from build123d import *

# Parameters (mm, degrees)
BOSS_EXTRUDE1_DEPTH = 50.8
SKETCH2_R           = 3.175
CUT_EXTRUDE1_DEPTH  = 64.5
SKETCH3_R           = 5.08
CUT_EXTRUDE2_DEPTH  = 19.05


with BuildPart() as part:
    # Sketch1 → Boss-Extrude1 (new body)
    with BuildSketch(Plane.XY):
        with BuildLine():
            Line((0, 101.6), (0, 114.3))
            ThreePointArc((0, 114.3), (-63.5, 50.8), (0, -12.7))
            Line((0, -12.7), (0, 0))
            ThreePointArc((0, 0), (-50.8, 50.8), (0, 101.6))
        make_face()
    extrude(amount=BOSS_EXTRUDE1_DEPTH)

    # Sketch2 → Cut-Extrude1 (cut, through all)
    with BuildSketch(Plane(origin=(0, 0, 0), x_dir=(0, 0, -1), z_dir=(1, 0, 0))):
        with Locations((-44.45, 107.95)):
            Circle(SKETCH2_R)
        with Locations((-6.35, 107.95)):
            Circle(SKETCH2_R)
        with Locations((-6.35, -6.35)):
            Circle(SKETCH2_R)
        with Locations((-44.45, -6.35)):
            Circle(SKETCH2_R)
    extrude(amount=-CUT_EXTRUDE1_DEPTH, mode=Mode.SUBTRACT)

    # Sketch3 → Cut-Extrude2 (cut)
    with BuildSketch(Plane(origin=(-38.1, 0, 0), x_dir=(0, 0, -1), z_dir=(1, 0, 0))):
        with Locations((-44.45, 107.95)):
            Circle(SKETCH3_R)
        with Locations((-6.35, 107.95)):
            Circle(SKETCH3_R)
        with Locations((-6.35, -6.35)):
            Circle(SKETCH3_R)
        with Locations((-44.45, -6.35)):
            Circle(SKETCH3_R)
    extrude(amount=CUT_EXTRUDE2_DEPTH, mode=Mode.SUBTRACT)


solid = part.part
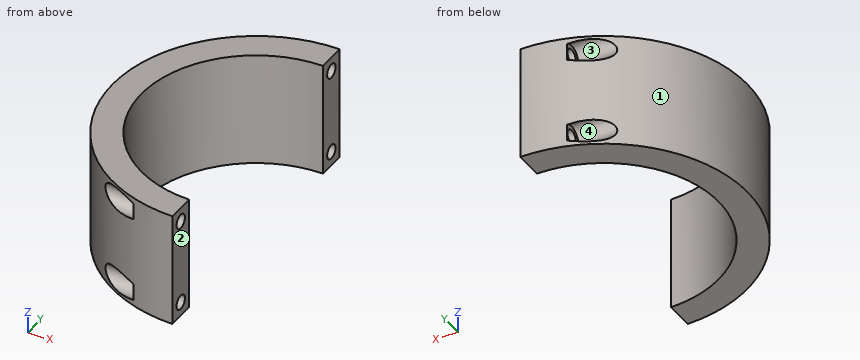
Design review of the part built by this model. Coordinates are the model's own, in mm. Face numbers are marked on the shaded views. Give positions to 0.01 mm unless a question says otherwise; leave off trailing zeros. Order: outer loops, then holes, each group sorted by start corner. A loop starts at its lowest first (then second) coordinate and runs counter-clockwise, first axis right, second up. Notation, with made-up numbers: (30.5, 44.25) - (53.5, 44.25) arc R9 ccw to (53.5, 59.25) - close; hole circle Ø1 at (-16, 9.5). An arc over 180 degrees is marked (long way). Use CSV: the item, a comma, the result in double quotes. Start each with the question number.
Q1. For line 1 (Z direction, x = -25, y = -6); line 2 (Y direction, x = -7.25, z = 44.45) (3 decimals); line 3 (Y direction, x = -13, z = 5), list the stretches that pass through material, from the lowest coordinate up.
Q2. Take a section at C-C (x = -21). State the section outline as (y, z) points, and give its area (3 significant figures).
Q3. Take a section at A-A (z = 6.35). State the section outline as (x, y) points (3 decimals).
Q4. For P1, Ø8, axis at y = 88, z = 7.5, coming from the -X side; P2, Ø10, axis at y = -6.35, z = 6.35, coming from the -X side; P3, Ø10, axis at x = -21, z = 8.5, coming from the +Y side; P4, Ø6, axis at y = 107.95, z = 6.35, coming from the -X side, all flat-tipped, find the tip position at first contact; note any pin that passes through.
Q5. Take a section at D-D (y = 107.95). State the section outline as (x, z) points (3 decimals).
Q6. Take a section at B-B (x = -8.5). State the section outline as (y, z) points (3 decimals).
Q7. Draft analysis for pull direction Y (two halves, no side actions). For the marked faces 1, 2, 3 and 4, state which applies: pulls with the +Y half, pulls with the -Y half, needs draft (parallel to the pull), parting line crosses it, or undercut.
Calculated:
1,line 1,"z = 0 to 1.28, 11.42 to 39.38, 49.52 to 50.8"
1,line 2,"y = -12.285 to -9.525, -3.175 to 0.52, 101.08 to 104.775, 111.125 to 113.885"
1,line 3,"y = -11.36 to -9.22, -3.48 to 1.69, 99.91 to 105.08, 110.82 to 112.96"
2,outline,"(-9.13, 0) - (4.54, 0) - (4.54, 50.8) - (-9.13, 50.8) - (-9.13, 48.7) arc R5.08 cw (long way) to (-9.13, 40.2) - (-9.13, 10.6) arc R5.08 cw (long way) to (-9.13, 2.1) - close; (97.06, 0) - (110.73, 0) - (110.73, 2.1) arc R5.08 cw (long way) to (110.73, 10.6) - (110.73, 40.2) arc R5.08 cw (long way) to (110.73, 48.7) - (110.73, 50.8) - (97.06, 50.8) - close"
2,area,"1,120 mm²"
3,outline,"(-36.345, -1.27) - (-19.05, -1.27) - (-19.05, -3.175) - (0, -3.175) - (0, 0) arc R50.8 cw to (0, 101.6) - (0, 104.775) - (-19.05, 104.775) - (-19.05, 102.87) - (-36.345, 102.87) arc R63.5 ccw to start; (-19.05, -9.775) arc R63.5 ccw to (0, -12.7) - (0, -9.525) - (-19.05, -9.525) - close; (-19.05, 111.125) - (0, 111.125) - (0, 114.3) arc R63.5 ccw to (-19.05, 111.375) - close"
4,P1,"stops at x = -54.13"
4,P2,"stops at x = -19.05"
4,P3,"stops at y = 112.25"
4,P4,"passes through"
5,outline,"(-27.679, 0) - (0, 0) - (0, 3.175) - (-19.05, 3.175) - (-19.05, 1.27) - (-27.679, 1.27) - close; (-27.679, 11.43) - (-19.05, 11.43) - (-19.05, 9.525) - (0, 9.525) - (0, 41.275) - (-19.05, 41.275) - (-19.05, 39.37) - (-27.679, 39.37) - close; (-27.679, 49.53) - (-19.05, 49.53) - (-19.05, 47.625) - (0, 47.625) - (0, 50.8) - (-27.679, 50.8) - close"
6,outline,"(-12.129, 0) - (0.716, 0) - (0.716, 50.8) - (-12.129, 50.8) - close; (100.884, 0) - (113.729, 0) - (113.729, 50.8) - (100.884, 50.8) - close; hole circle Ø6.35 at (-6.35, 6.35); hole circle Ø6.35 at (-6.35, 44.45); hole circle Ø6.35 at (107.95, 6.35); hole circle Ø6.35 at (107.95, 44.45)"
7,face 1,"parting line crosses it"
7,face 2,"needs draft"
7,face 3,"undercut"
7,face 4,"undercut"
